The listing builds one solid part. Answer for the finished solid, in the listing's coordinates (mm). A direction names the side the tool comes from. Coordinates: 2 decimals unless noted, no trailing zeros. Write each loop counter-clockwise with the first axis right and the second up, starting at its lowest first coordinate (ties: lowest second). Pieces come first, ordered by that corner, then holes.
```python
from build123d import *

# Parameters (mm, degrees)
F0_R     = 76.2
F1_DEPTH = 25.4
F3_DEPTH = 25.4
F4_COUNT = 20


with BuildPart() as f1:
    # F0 (on Front) → F1 (new body)
    with BuildSketch(Plane.XZ):
        Circle(F0_R)
    extrude(amount=F1_DEPTH)

    # F2 (on face) → F3 (join, through all)
    with BuildSketch(Plane.XZ.offset(25.4)):
        Polygon((7.153107319, 99.4136035442), (-6.2727834728, 75.941373358), (7.153107319, 75.8635159723), align=None)
    extrude(amount=-F3_DEPTH)

    # F4: F1 ×20 about axis
    f4_axis = Axis((0, 0, 0), (0, 1, 0))


with BuildPart() as f1_1:
    add(f1.part)
    for i in range(1, F4_COUNT):
        add(f1.part.rotate(f4_axis, i * 360 / F4_COUNT))


solid = f1_1.part
```
(1) Each of these flat-tipped pins is pushed along its axis until it touches: pin 1 (10 mm diameter, centred on x = -35, z = 34.5, fed in from +Y); pin 2 (12 mm diameter, centred on x = 88.5, y = -9, fed in from -Z); pin 3 (5 mm diameter, centred on y = -10.5, z = -26.5, fed in from +X); pin 4 (3 mm diameter, centred on x = -46, y = -21, fed in from -Z). Where does it stop, or does it pass through?
(2) Section A-A, the plane x = 2.5 is taken. Write down the section's boundary in (y, z).
(3) Section B-B, the plane z = -1 is taken. Write down the section's boundary in (x, y).
(4) Find the intervals of material crossed by probe 1 along Z at (x, y) = (-66, -14.5); probe 2 along Z at (x, y) = (-68.5, -11); probe 3 along X at (y, z) = (-13.25, 88), in increasing order.
(5) Which of the six approach directions +Z, -Z, +X, -X, +Y, -Y give full straight-line access (tool end or side, diameter ignored) to faces 1 (the flat face through (-52.06, -12.88, -70.75)), 2 (the flat face through (87, -13, -7.153)), 3 (the cylindrical face through (12.43, -12.52, 75.18))?
Solution:
1. pin 1: stops at y = 0
1. pin 2: stops at z = -37.52
1. pin 3: stops at x = 84.6
1. pin 4: stops at z = -68.7
2. outline: (-25.4, -82.54) - (0, -82.54) - (0, 91.28) - (-25.4, 91.28) - close
3. outline: (-85.16, -25.4) - (88.66, -25.4) - (88.66, 0) - (-85.16, 0) - close
4. probe 1: z = -50.61 to -39.11, -38.08 to 38.08, 41.51 to 56.79
4. probe 2: z = -50.89 to -40.93, -33.38 to 33.38, 47.06 to 58.61
4. probe 3: x = -25.74 to -21.07, 0.62 to 7.15, 32.75 to 36.11
5. face 1: -Z, +Y, -Y
5. face 2: +X, +Y, -Y
5. face 3: +Z, +Y, -Y
